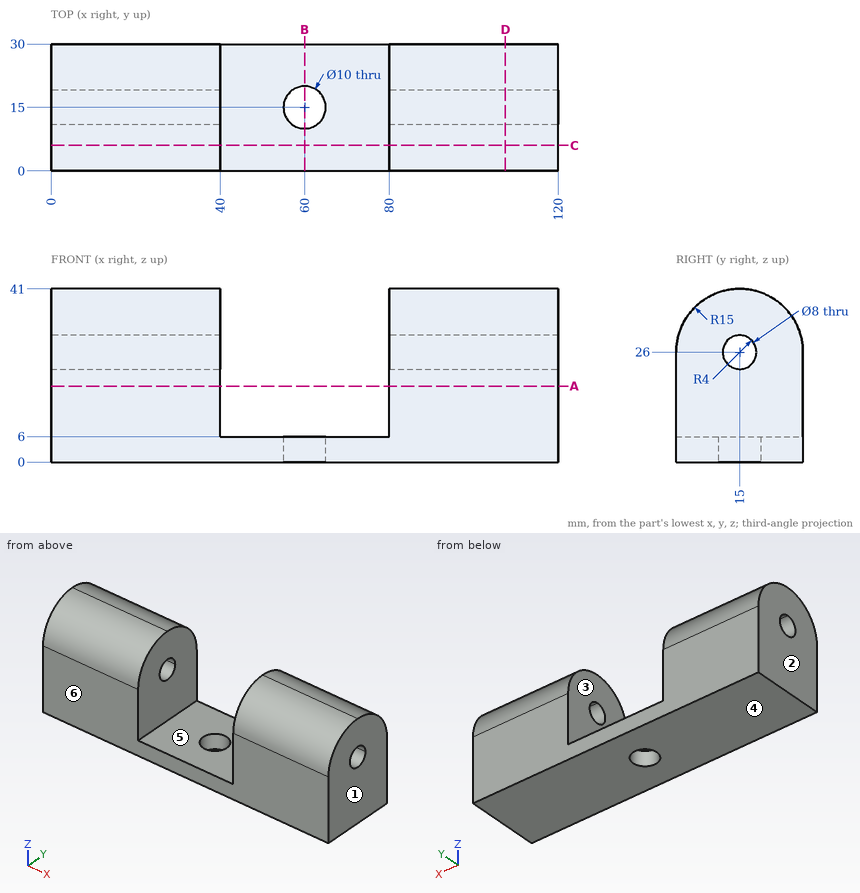
The figure shows three views and two pictorial views of one solid part (mm, origin at its lowest corner). Answer the questions. A direction names the side the tool comes from. Round coordinates to 2 decimals unless told otherwise and drop trailing zeros. Order: outer loops, then holes, each group sorted by start corner. A loop starts at its lowest first (then second) coordinate and runs counter-clockwise, first axis right, second up. Notation, with made-up numbers: (-19, -1) -> (12, -1) arc R35 cw to (12, 31) -> close; hole circle Ø2 at (42.25, 52.5). An arc over 180 degrees is marked (long way). Put each result on its own line as item: value.
Q1. Determine the mould class of the marked faces 1, 2, 3 and 4 for opening direction X: pulls with the +X half, pulls with the -X half, needs draft (parallel to the pull), parting line crosses it, or undercut.
Results list:
face 1: pulls with the +X half
face 2: pulls with the -X half
face 3: undercut
face 4: needs draft
Q2. Consider line 1 along X through (y, z) = (8.5, 30); line 2 along Y through (x, z) = (60, 4.15); line 3 along Y through (x, z) = (102, 26). Determine where each line is inside the solid, lowest interval first.
Results list:
line 1: 0 to 40, 80 to 120
line 2: 0 to 10, 20 to 30
line 3: 0 to 11, 19 to 30
Q3. Which of the six approach directions +Z, -Z, +X, -X, +Y, -Y give full straight-line access (tool end or side, diameter ignored) to the marked faces 5 and 6?
Results list:
face 5: +Z, +Y, -Y
face 6: +Z, -Z, +X, -X, -Y
Q4. Section D-D, the plane x = 107.5 is taken. Write down the section's boundary in (y, z).
Results list:
outline: (0, 0) -> (30, 0) -> (30, 26) arc R15 ccw to (15, 41) arc R15 ccw to (0, 26) -> close; hole circle Ø8 at (15, 26)
Q5. Section B-B, the plane x = 60 is taken. Write down the section's boundary in (y, z).
Results list:
outline: (0, 0) -> (10, 0) -> (10, 6) -> (0, 6) -> close; (20, 0) -> (30, 0) -> (30, 6) -> (20, 6) -> close
Q6. Each of these flat-tipped pins is pushed along its axis until it touches: P1, Ø10, axis at x = 76.5, z = 33.5, coming from the -Y side; P2, Ø12, axis at x = 18.5, z = 35.5, coming from the -Y side; P3, Ø16, axis at x = 60, y = 15, coming from the +Z side. Where does it stop, or does it pass through?
Results list:
P1: y = 0.52
P2: y = 0.41
P3: z = 6
Q7. Section C-C, the plane y = 6 is taken. Write down the section's boundary in (x, z).
Results list:
outline: (0, 0) -> (120, 0) -> (120, 38) -> (80, 38) -> (80, 6) -> (40, 6) -> (40, 38) -> (0, 38) -> close
Q8. Section A-A, the plane z = 18 is taken. Write down the section's boundary in (x, y), and give its area (3 significant figures).
Results list:
outline: (0, 0) -> (40, 0) -> (40, 30) -> (0, 30) -> close; (80, 0) -> (120, 0) -> (120, 30) -> (80, 30) -> close
area: 2,400 mm^2
